from build123d import *

# Parameters (mm, degrees)
SKETCH1_R           = 3.1877
SKETCH1_R_2         = 11.2776
BOSS_EXTRUDE1_DEPTH = 6.35
SKETCH2_W           = 5.08
SKETCH2_H           = 30.1625
BOSS_EXTRUDE2_DEPTH = 6.35
FILLET1_R           = 6.35


with BuildPart() as part:
    # Sketch1 → Boss-Extrude1 (new body)
    with BuildSketch(Plane.XY):
        Polygon((-38.1, 15.08125), (59.69, 15.08125), (75.565, 9.525), (75.565, -9.525), (59.69, -15.08125), (-38.1, -15.08125), (-53.975, -9.525), (-53.975, 9.525), align=None)
        Circle(SKETCH1_R, mode=Mode.SUBTRACT)
        with Locations((-38.1, 0)):
            Circle(SKETCH1_R_2, mode=Mode.SUBTRACT)
        with Locations((59.69, 0)):
            Circle(SKETCH1_R_2, mode=Mode.SUBTRACT)
    extrude(amount=BOSS_EXTRUDE1_DEPTH)

    # Sketch2 → Boss-Extrude2 (add)
    with BuildSketch(Plane.XY.offset(6.35)):
        with Locations((-15.367, 0)):
            Rectangle(SKETCH2_W, SKETCH2_H)
        with Locations((15.367, 0)):
            Rectangle(SKETCH2_W, SKETCH2_H)
    extrude(amount=BOSS_EXTRUDE2_DEPTH)

    # Fillet1
    fillet1_edges = [part.edges().sort_by_distance(p)[0] for p in [
        (-17.907, 0, 6.35),
        (17.907, 0, 6.35),
    ]]
    fillet(fillet1_edges, radius=FILLET1_R - 0.0001)  # a hair under: the kernel refuses the full size


solid = part.part
Model file for the job. Use its own axes, mm. A direction names the side the tool comes from. Coordinates: 2 decimals unless noted, no trailing zeros. Order: outer loops, then holes, each group sorted by start corner. A loop starts at its lowest first (then second) coordinate and runs counter-clockwise, first axis right, second up. Notation, with made-up numbers: (16, 78.5) -> (34, 78.5) arc R20 cw to (34, 86.5) -> close; hole circle Ø2 at (-19, -20.5). An arc over 180 degrees is marked (long way). Return JSON: item names as keys, results as strings. Group by question number.
Item 1: Flat gauge pins, fed straight in: P1, Ø13, axis at x = 4, y = 4.5, coming from the +Z side; P2, Ø5, axis at y = 1.5, z = 10, coming from the -X side. Where does each tip first touch, or does it go through?
Item 2: Pull direction X, two halves, no side cores. Call faces 4 (the flat face through (-46.149, 12.264, 3.131)), 5 (the flat face through (12.827, 0, 9)), 6 (the flat face through (67.52, 12.34, 3.13)), 7 (the cylindrical face through (70.447, 3.387, 3.131)): pulls with the +X half, pulls with the -X half, needs draft (parallel to the pull), parting line crosses it, or undercut.
Item 3: Saw through at A-A on x = 0. Write the cut outline in (y, z), then the cut area to 3 significant figures.
Item 4: Tool access for faces 1 (the flat face through (-29, 7, 6.35)), 2 (the flat face through (-12.827, 0, 9)), 3 (the flat face through (45, 0, 6.35)): list every direction of +Z, -Z, +X, -X, +Y, -Y with a clear straight run to the whole face (end or side of a thin tool).
Item 5: Saw through at C-C on z = 10.25. Write the cut outline in (x, y), then the cut area to 3 significant figures.
Item 6: Wall check: line 1 along Y through (x, z) = (59.69, 3.25); line 2 along Y through (x, z) = (0, 2.5); line 3 along X through (y, z) = (1, 2) (3 decimals). Give the ranges that are in metal, low to high. Write a range as [from, to].
Item 7: Saw through at B-B on y = 0. State how many separate pieces and enclosed holes the cut face has, then the cut area to 3 significant figures.
Values found:
{
 "1": {"P1": "stops at z = 6.35", "P2": "stops at x = -20.61"},
 "2": {"face 4": "pulls with the -X half", "face 5": "undercut", "face 6": "pulls with the +X half", "face 7": "undercut"},
 "3": {"outline": "(-15.08, 0) -> (-3.19, 0) -> (-3.19, 6.35) -> (-15.08, 6.35) -> close; (3.19, 0) -> (15.08, 0) -> (15.08, 6.35) -> (3.19, 6.35) -> close", "area": "151 mm2"},
 "4": {"face 1": "+Z, -X, +Y, -Y", "face 2": "+Z, +Y, -Y", "face 3": "+Z, +X, +Y, -Y"},
 "5": {"outline": "(-18.4, -15.08) -> (-12.83, -15.08) -> (-12.83, 15.08) -> (-18.4, 15.08) -> close; (12.83, -15.08) -> (18.4, -15.08) -> (18.4, 15.08) -> (12.83, 15.08) -> close", "area": "336 mm2"},
 "6": {"line 1": "y = [-15.08, -11.28], [11.28, 15.08]", "line 2": "y = [-15.08, -3.19], [3.19, 15.08]", "line 3": "x = [-53.975, -49.333], [-26.867, -3.027], [3.027, 48.457], [70.923, 75.565]"},
 "7": {"separate pieces": "4", "enclosed holes": "0", "area": "577 mm2"}
}
